```python
from build123d import *

# Parameters (mm, degrees)
BOSS_EXTRUDE1_DEPTH = 1.5875


with BuildPart() as part:
    # Sketch2 → Boss-Extrude1 (new, symmetric)
    with BuildSketch(Plane.XY):
        with BuildLine():
            Line((0, -93.726), (0, -78.486))
            ThreePointArc((0, -78.486), (45.497909529, -102.143988159), (95.5675, -113.225336692))
            ThreePointArc((95.5675, -113.225336692), (247.168367606, -119.728946816), (398.720709803, -112.17861051))
            ThreePointArc((398.720709803, -112.17861051), (494.586291489, -94.575813643), (588.578984507, -68.779653684))
            Line((588.578984507, -68.779653684), (590.864339182, -81.353629169))
            ThreePointArc((590.864339182, -81.353629169), (496.464017617, -107.14437724), (400.203586993, -124.765753286))
            ThreePointArc((400.203586993, -124.765753286), (247.115945932, -132.400573942), (93.98, -125.805242584))
            ThreePointArc((93.98, -125.805242584), (45.058861039, -115.423125179), (0, -93.726))
        make_face()
    extrude(amount=BOSS_EXTRUDE1_DEPTH, both=True)


solid = part.part
```
Here's how the part is built. I have some questions about the finished solid (model axes, mm). A direction names the side the tool comes from. Give positions to 0.01 mm unless a question says otherwise; leave off trailing zeros. Loops run counter-clockwise (first coordinate to the right, second up) from the corner with the lowest first, then second, coordinate; pieces in that order, holes last. Notation, with made-up numbers: (73.5, 53.5) -> (86.5, 53.5) arc R8 ccw to (86.5, 61.5) -> close; hole circle Ø5 at (-11.75, 12.25). An arc over 180 degrees is marked (long way). Use one line per item in the form item = value. Start each with the question number.
1) Please list where these lines run through material, in increasing order: line 1 along Y through (x, z) = (260, -0.25); line 2 along Y through (x, z) = (543.5, -0.05).
2) Imagine slicing it at C-C (x = 100.5). Please give me the cut outline in (y, z), then the cut area to 3 significant figures.
3) Which directions (+Z, -Z, +X, -X, +Y, -Y) give clear straight access to the entire face, cutting with the end or side of a thin tool? Please do faces 4 (the face through (297, -122, -1.588)), 5 (the face through (493.26, -94.88, 0.02)).
4) Thinking about a two-plate mould opening in X: for faces 1 (the face through (44.822, -101.897, 0.022)), 2 (the face through (297, -122, 1.588)), 3 (the face through (45.723, -115.649, 0.022)), which applies, +X half, -X half, draft (parallel to the pull), parting line (faces both ways), or undercut?
5) Imagine slicing it at B-B (x = 213). Please give me the cut outline in (y, z), then the cut area to 3 significant figures.
6) Imagine slicing it at A-A (z = 0.7). Please give me the cut outline in (x, y), then the cut area to 3 significant figures.
Check values:
q1.line_1 = -132.31 to -119.63
q1.line_2 = -95.38 to -82.24
q2.outline = (-126.38, -1.59) -> (-113.66, -1.59) -> (-113.66, 1.59) -> (-126.38, 1.59) -> close
q2.area = 40.4 mm^2
q3.face_4 = -Z, +X, -X, +Y, -Y
q3.face_5 = +Z, -Z, +Y
q4.face_1 = undercut
q4.face_2 = draft
q4.face_3 = -X half
q5.outline = (-132.16, -1.59) -> (-119.49, -1.59) -> (-119.49, 1.59) -> (-132.16, 1.59) -> close
q5.area = 40.2 mm^2
q6.outline = (0, -93.73) arc R209.19 ccw to (93.98, -125.81) arc R1651 ccw to (400.2, -124.77) arc R1143 ccw to (590.86, -81.35) -> (588.58, -68.78) arc R1130.33 cw to (398.72, -112.18) arc R1638.33 cw to (95.57, -113.23) arc R196.52 cw to (0, -78.49) -> close
q6.area = 7,630 mm^2
